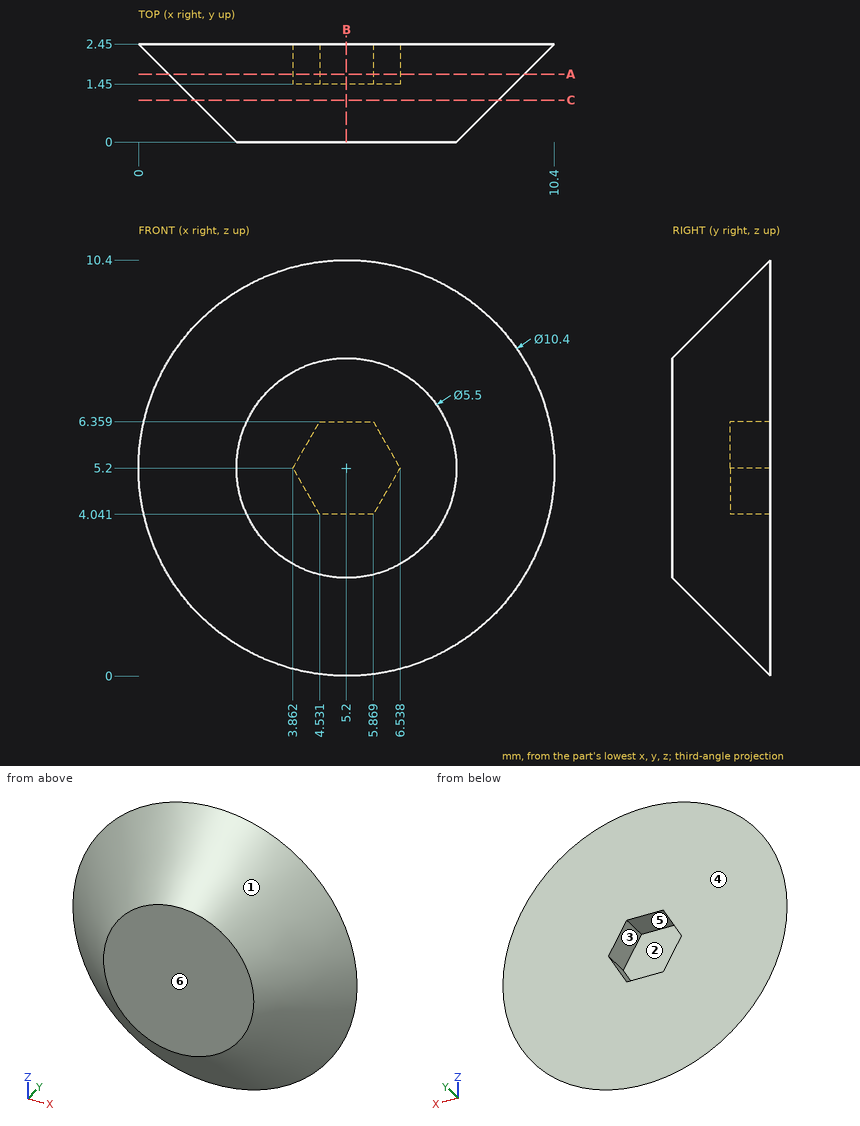
Geometry: see drawing. Coordinates: mm, zero at the bounding-box minimum. A direction names the side the tool comes from. Round coordinates to 2 decimals unless told otherwise and drop trailing zeros. Write each loop counter-clockwise with the first axis right and the second up, starting at its lowest first coordinate (ties: lowest second). Pieces come first, ordered by that corner, then holes.
Item 1: Mould query, pull axis Z, two halves, no side actions, for the marked faces 1, 2, 3 and 4. Classes: +Z half, -Z half, draft (parallel to the pull), parting line (faces both ways), or undercut.
Item 2: Section query A-A (y = 1.7). Return loops of the section in (x, z).
Item 3: Set-up query: the marked faces 5 and 6. Return all of +Z, -Z, +X, -X, +Y, -Y with unobstructed straight access to the full face (end or side cutting, diameter ignored); none if empty.
Item 4: Pin query (flat end, axial travel): P1, Ø2, axis at x = 5.5, z = 9, coming from the -Y side; P2, Ø0.5, axis at x = 5.5, y = 2, coming from the +Z side; P3, Ø0.5, axis at x = 5.5, y = 2, coming from the -Z side. Return the tip coordinate at first contact, or that it passes through.
Item 5: Section query C-C (y = 1.05). Return loops of the section in (x, z), plus the area to 3 significant figures.
Item 6: Section query B-B (x = 5.2). Return loops of the section in (y, z).
Item 7: Material intervals for L1, parallel to X at y = 1.7, z = 8.5 (1 decimal); L2, parallel to Z at x = 4.75, y = 1; L3, parallel to Z at x = 7.5, y = 1.9, sorted ascending.
Completed:
1. face 1: parting line
1. face 2: undercut
1. face 3: undercut
1. face 4: draft
2. outline: circle Ø8.9 at (5.2, 5.2); hole (3.86, 5.2) - (4.53, 4.04) - (5.87, 4.04) - (6.54, 5.2) - (5.87, 6.36) - (4.53, 6.36) - close
3. face 5: +Y
3. face 6: +Z, -Z, +X, -X, -Y
4. P1: stops at y = 0.06
4. P2: stops at z = 10.19
4. P3: stops at z = 0.21
5. outline: circle Ø7.6 at (5.2, 5.2)
5. area: 45.4 mm2
6. outline: (0, 2.45) - (2.45, 0) - (2.45, 4.04) - (1.45, 4.04) - (1.45, 6.36) - (2.45, 6.36) - (2.45, 10.4) - (0, 7.95) - close
7. L1: x = 2.2 to 8.2
7. L2: z = 1.48 to 8.92
7. L3: z = 1.16 to 9.24
